from build123d import *

# Parameters (mm, degrees)
F1_DEPTH = 5
F3_DEPTH = 26
F4_R     = 15
F5_R     = 6


with BuildPart() as f1:
    # F0 (on Front) → F1 (new body)
    with BuildSketch(Plane.XZ):
        with BuildLine():
            Line((15.0000003353, -79.3999582529), (15.0000003353, 25.8973006904))
            Line((15.0000003353, 25.8973006904), (-14.9999996647, 25.8973006904))
            Line((-14.9999996647, 25.8973006904), (-14.9999996647, -79.3999582529))
            ThreePointArc((-14.9999996647, -79.3999582529), (3.353e-07, -64.3999582529), (15.0000003353, -79.3999582529))
        make_face()
        with BuildLine():
            ThreePointArc((-14.9999996647, -79.3999582529), (3.353e-07, -94.3999582529), (15.0000003353, -79.3999582529))
            Line((15.0000003353, -79.3999582529), (7.5000003353, -79.3999582529))
            ThreePointArc((7.5000003353, -79.3999582529), (3.353e-07, -86.8999582529), (-7.4999996647, -79.3999582529))
            Line((-7.4999996647, -79.3999582529), (-14.9999996647, -79.3999582529))
        make_face()
        with BuildLine():
            Line((7.5000003353, -79.3999582529), (15.0000003353, -79.3999582529))
            ThreePointArc((15.0000003353, -79.3999582529), (3.353e-07, -64.3999582529), (-14.9999996647, -79.3999582529))
            Line((-14.9999996647, -79.3999582529), (-7.4999996647, -79.3999582529))
            ThreePointArc((-7.4999996647, -79.3999582529), (3.353e-07, -71.8999582529), (7.5000003353, -79.3999582529))
        make_face()
    extrude(amount=F1_DEPTH)

    # F2 (on Top) → F3 (join)
    with BuildSketch(Plane.XY):
        with BuildLine():
            ThreePointArc((11.6990586319, 69.4567795833), (37.8389339862, 34.4401238089), (11.9304887253, -0.7481090158))
            Line((11.9304887253, -0.7481090158), (14.999749139, -4.999996163))
            ThreePointArc((14.999749139, -4.999996163), (42.8296580573, 35.2079426128), (13.3109600907, 74.1929223018))
            Line((13.3109600907, 74.1929223018), (11.6990586319, 69.4567795833))
        make_face()
    extrude(amount=F3_DEPTH)

    # F4
    f4_edges = [f1.edges().sort_by_distance(p)[0] for p in [
        (-15, -2.5, 25.897301),
    ]]
    fillet(f4_edges, radius=F4_R)

    # F5
    f5_edges = [f1.edges().sort_by_distance(p)[0] for p in [
        (15, -2.499954, 0),
    ]]
    fillet(f5_edges, radius=F5_R)


solid = f1.part
Can you work these out from the model? Positions are in its coordinate system, mm. A direction names the side the tool comes from. Coordinates: 2 decimals unless noted, no trailing zeros. Write each loop counter-clockwise with the first axis right and the second up, starting at its lowest first coordinate (ties: lowest second). Pieces come first, ordered by that corner, then holes. Notation, with made-up numbers: (29.5, -29) - (62.5, -29) arc R16 ccw to (62.5, -19) - close; hole circle Ø3 at (10.5, 3). An arc over 180 degrees is marked (long way). Return JSON: item names as keys, results as strings. Group by question number.
Item 1: If we section it at A-A (z = -84.5): Write out the boundary of the cut face in (x, y).
Item 2: If we section it at B-B (x = 4.5): Write out the boundary of the cut face in (y, z), then the cut area to 3 significant figures.
Item 3: Which directions (+Z, -Z, +X, -X, +Y, -Y) give clear straight access to the entire face, cutting with the end or side of a thin tool? Please do faces 4 (the face through (15, -2, -39)), 5 (the face through (0, -5, -33)).
Item 4: Please list where these lines run through material, in increasing order: probe 1 along Y at (x, z) = (-10.5, -32); probe 2 along Z at (x, y) = (31.5, 56); probe 3 along X at (y, z) = (28, 9.5).
Item 5: We'd pull the mould along X, two halves only. Please class faces 1 (the face through (-0.976, -2.465, -86.836)), 2 (the face through (-15, -2, -34)), 3 (the face through (8, -2, 25.897)): pulls with the +X half, pulls with the -X half, needs draft (parallel to the pull), parting line crosses it, or undercut.
Item 6: I'm going to push flat-ended pins straight in: pin 1 Ø4 at (x, z) = (-2.5, -72.5) entering from -Y; pin 2 Ø18 at (x, z) = (7.5, -47.5) entering from +Y; pin 3 Ø25 at (x, y) = (29, 22) entering from -Z; pin 4 Ø2.5 at (x, y) = (9.5, -1.5) entering from +Z. Where does each tip first touch, or does it pass through?
Item 7: If we section it at D-D (y = 5): Write out the boundary of the cut face in (x, z), then the cut area to 3 significant figures.
Return value:
{
 "1": {"outline": "(-14.11, -5) - (-5.5, -5) - (-5.5, 0) - (-14.11, 0) - close; (5.5, -5) - (14.11, -5) - (14.11, 0) - (5.5, 0) - close"},
 "2": {"outline": "(-5, -93.71) - (0, -93.71) - (0, -85.4) - (-5, -85.4) - close; (-5, -73.4) - (0, -73.4) - (0, 25.9) - (-5, 25.9) - close", "area": "538 mm^2"},
 "3": {"face 4": "-Z, +X, +Y, -Y", "face 5": "+Z, -Z, +X, -X, -Y"},
 "4": {"probe 1": "y = -5 to 0", "probe 2": "z = 0 to 26", "probe 3": "x = 37.29 to 42.36"},
 "5": {"face 1": "undercut", "face 2": "pulls with the -X half", "face 3": "needs draft"},
 "6": {"pin 1": "stops at y = -5", "pin 2": "stops at y = 0", "pin 3": "stops at z = 0", "pin 4": "stops at z = 25.9"},
 "7": {"outline": "(23.2, 0) - (30.79, 0) - (30.79, 26) - (23.2, 26) - close", "area": "197 mm^2"}
}
